Design review of the part built by this model. Coordinates are the model's own, in mm. A direction names the side the tool comes from. Give positions to 0.01 mm unless a question says otherwise; leave off trailing zeros. Loops run counter-clockwise (first coordinate to the right, second up) from the corner with the lowest first, then second, coordinate; pieces in that order, holes last. Notation, with made-up numbers: (68, 49) - (113, 49) arc R16 ccw to (113, 62) - close; hole circle Ø4 at (-27.75, -15.75). An arc over 180 degrees is marked (long way). One line per item, written item: value. Start each with the question number.
```python
from build123d import *

# Parameters (mm, degrees)
SKETCH2_R           = 7.5
BOSS_EXTRUDE1_DEPTH = 3.5
SKETCH3_R           = 4.5
BOSS_EXTRUDE2_DEPTH = 15
FILLET1_R           = 1
FILLET2_R           = 0.5


with BuildPart() as part:
    # Sketch2 → Boss-Extrude1 (new body)
    with BuildSketch(Plane(origin=(0, 0, 0), x_dir=(1, 0, 0), z_dir=(0, 1, 0))):
        Circle(SKETCH2_R)
    extrude(amount=BOSS_EXTRUDE1_DEPTH)

    # Sketch3 → Boss-Extrude2 (add)
    with BuildSketch(Plane(origin=(0, 3.5, 0), x_dir=(1, 0, 0), z_dir=(0, 1, 0))):
        Circle(SKETCH3_R)
    extrude(amount=BOSS_EXTRUDE2_DEPTH)

    # Fillet1
    fillet1_edges = [part.edges().sort_by_distance(p)[0] for p in [
        (-7.5, 0, 0),
    ]]
    fillet(fillet1_edges, radius=FILLET1_R)

    # Fillet2
    fillet2_edges = [part.edges().sort_by_distance(p)[0] for p in [
        (-7.5, 3.5, 0),
    ]]
    fillet(fillet2_edges, radius=FILLET2_R)


solid = part.part
```
(1) Take a section at C-C on y = 14. State the section outline as (x, z) points.
(2) Machinability: for faces 1 (the cylindrical face through (-7.493, 1.986, -0.33)), 2 (the cylindrical face through (-0.59, 10.9, -4.46)), which of the approach directions +Z, -Z, +X, -X, +Y, -Y give a long, thin tool a straight path to every point of the face, cutting with its end or side? Answer none if there is none.
(3) To check wall thickness, follow L1, parallel to Y at x = 1, z = 6; L2, parallel to X at y = 14.75, z = -2. State the ranges of each line that lie inside material, in increasing order. Write a range as from..to.
(4) Take a section at B-B on x = 0. State the section outline as (y, z) points, and give its area (3 significant figures).
(5) For pin 1 Ø1.5 at (y, z) = (7.5, -2) entering from +X; pin 2 Ø3 at (x, y) = (-5.5, 3.5) entering from +Z; pin 3 Ø2 at (x, z) = (-3.5, -5) entering from +Y, all flat-tipped, find the tip position at first contact; note any pin that passes through.
(6) Take a section at A-A on z = 0. State the section outline as (x, y) points.
Here are the results:
1. outline: circle Ø9 at (0, 0)
2. face 1: +Y, -Y
2. face 2: +Y
3. L1: 0..3.5
3. L2: -4.03..4.03
4. outline: (0, -6.5) arc R1 ccw to (1, -7.5) - (3, -7.5) arc R0.5 ccw to (3.5, -7) - (3.5, -4.5) - (18.5, -4.5) - (18.5, 4.5) - (3.5, 4.5) - (3.5, 7) arc R0.5 ccw to (3, 7.5) - (1, 7.5) arc R1 ccw to (0, 6.5) - close
4. area: 187 mm²
5. pin 1: x = 4.32
5. pin 2: z = 6.3
5. pin 3: y = 3.5
6. outline: (-7.5, 1) arc R1 ccw to (-6.5, 0) - (6.5, 0) arc R1 ccw to (7.5, 1) - (7.5, 3) arc R0.5 ccw to (7, 3.5) - (4.5, 3.5) - (4.5, 18.5) - (-4.5, 18.5) - (-4.5, 3.5) - (-7, 3.5) arc R0.5 ccw to (-7.5, 3) - close
